Check sheet for the modelled part. Datum: model origin and axes. Units: mm. A direction names the side the tool comes from. Give positions to 0.01 mm unless a question says otherwise; leave off trailing zeros. Order: outer loops, then holes, each group sorted by start corner. A loop starts at its lowest first (then second) coordinate and runs counter-clockwise, first axis right, second up.
```python
from build123d import *

# Parameters (mm, degrees)
F0_W     = 112
F0_H     = 51
F1_DEPTH = 57
F2_W     = 74
F2_H     = 16
F3_DEPTH = 38
F4_W     = 19
F4_H     = 19
F5_DEPTH = 57.001
F6_W     = 36
F6_H     = 19
F7_DEPTH = 19
F9_DEPTH = 16


with BuildPart() as f1:
    # F0 (on Front) → F1 (new body)
    with BuildSketch(Plane.XZ):
        with Locations((56, 25.5)):
            Rectangle(F0_W, F0_H)
    extrude(amount=F1_DEPTH)

    # F2 (on face) → F3 (cut)
    with BuildSketch(Plane.XZ.offset(57)):
        with Locations((56, 43)):
            Rectangle(F2_W, F2_H)
    extrude(amount=-F3_DEPTH, mode=Mode.SUBTRACT)

    # F4 (on face) → F5 (cut, through all)
    with BuildSketch(Plane.XZ.offset(57)):
        with Locations((28.5, 25.5)):
            Rectangle(F4_W, F4_H)
        with Locations((83.5, 25.5)):
            Rectangle(F4_W, F4_H)
    extrude(amount=-F5_DEPTH, mode=Mode.SUBTRACT)

    # F6 (on face) → F7 (cut)
    with BuildSketch(Plane.XZ.offset(57)):
        with Locations((56, 25.5)):
            Rectangle(F6_W, F6_H)
    extrude(amount=-F7_DEPTH, mode=Mode.SUBTRACT)

    # F8 (on face) → F9 (cut)
    with BuildSketch(Plane(origin=(0, 0, 0), x_dir=(1, 0, 0), z_dir=(0, 0, -1))):
        with BuildLine():
            ThreePointArc((64, 38), (61.656854, 43.656854), (56, 46))
            ThreePointArc((56, 46), (50.343146, 32.343146), (64, 38))
        make_face()
    extrude(amount=-F9_DEPTH, mode=Mode.SUBTRACT)


solid = f1.part
```
(1) Tool access check on faces 5 (the face through (56, -35, 16)), 6 (the face through (56, -38, 26)), 7 (the face through (74, -19, 25)). Record the directions out of +Z, -Z, +X, -X, +Y, -Y that give a thin tool (end or side, any length) a straight path to the whole face; none if there is none.
(2) Sectioned sample at D-D (x = 43.5). Enter the section's corners in (y, z).
(3) Sectioned sample at C-C (y = -14). Enter the section's corners in (x, z), plus the area to 3 significant figures.
(4) Sectioned sample at A-A (z = 6). Enter the section's corners in (x, y), plus the area to 3 significant figures.
(5) Sectioned sample at B-B (z = 20.5). Enter the section's corners in (x, y).
(6) Release check for a two-part mould opening along X. For faces 1 (the face through (55, 0, 26)), 2 (the face through (38, -19, 25)), 3 (the face through (0, -28, 25)), 4 (the face through (112, -28, 25)) record: released by +X, released by -X, zero draft, split by the parting line, or undercut.
(7) Go/stop test with flat-tipped pins: P1, Ø1.5, axis at x = 63.5, y = -6, coming from the -Z side; P2, Ø9.5, axis at x = 48.5, y = -27.5, coming from the +Z side; P3, Ø17.5, axis at x = 60.5, z = 39, coming from the -Y side; P4, Ø9, axis at x = 54.5, y = -35.5, coming from the -Z side. Record where each tip stops, or that it passes through.
(8) Thickness scan on L1, parallel to X at y = -13, z = 30; L2, parallel to X at y = -38, z = 8.75; L3, parallel to Y at x = 56, z = 6.25. Record the ranges inside material, lowest first.
Values follow:
1. face 5: -Z
1. face 6: +Z, -Y
1. face 7: +Y, -Y
2. outline: (-57, 0) - (0, 0) - (0, 51) - (-19, 51) - (-19, 35) - (-38, 35) - (-38, 16) - (-57, 16) - close
3. outline: (0, 0) - (112, 0) - (112, 51) - (0, 51) - close; hole (19, 16) - (38, 16) - (38, 35) - (19, 35) - close; hole (74, 16) - (93, 16) - (93, 35) - (74, 35) - close
3. area: 4,990 mm2
4. outline: (0, -57) - (112, -57) - (112, 0) - (0, 0) - close; hole circle Ø16 at (56, -38)
4. area: 6,180 mm2
5. outline: (0, -57) - (19, -57) - (19, 0) - (0, 0) - close; (38, -38) - (74, -38) - (74, 0) - (38, 0) - close; (93, -57) - (112, -57) - (112, 0) - (93, 0) - close
6. face 1: zero draft
6. face 2: undercut
6. face 3: released by -X
6. face 4: released by +X
7. P1: stops at z = 0
7. P2: stops at z = 35
7. P3: stops at y = -38
7. P4: stops at z = 16
8. L1: x = 0 to 19, 38 to 74, 93 to 112
8. L2: x = 0 to 48, 64 to 112
8. L3: y = -57 to -46, -30 to 0
